The drawing under review shows one solid part. Ordinate dimensions are in mm from its lowest x, y, z. Give positions to 0.01 mm unless a question says otherwise; leave off trailing zeros. Loops run counter-clockwise (first coordinate to the right, second up) from the corner with the lowest first, then second, coordinate; pieces in that order, holes last. Notation, with made-up numbers: (43, -21) - (53, -21) arc R34 cw to (53, 15) - close; hole circle Ø11 at (-31.75, 80.25). An arc over 180 degrees is marked (long way). Write each question's results on one line, items separated by ' | '.
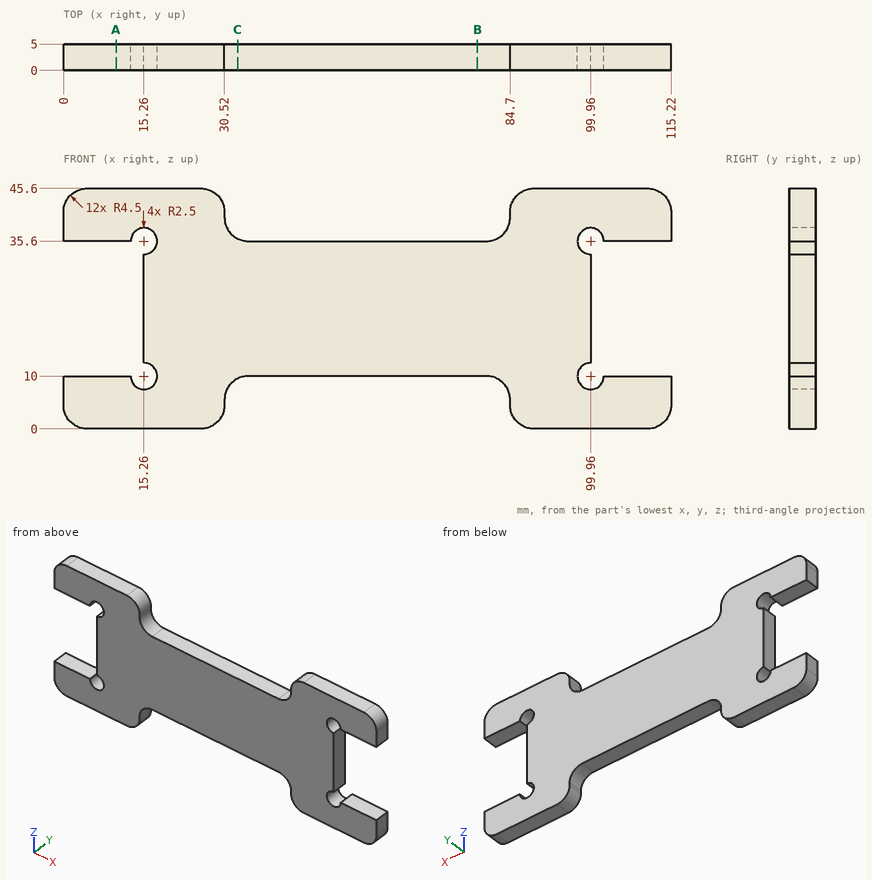
(1) Take a section at A-A on x = 10. Give the boundary of the cut face in (y, z), plus the area to 3 significant figures.
Answers below:
outline: (0, 0) - (5, 0) - (5, 10) - (0, 10) - close; (0, 35.6) - (5, 35.6) - (5, 45.6) - (0, 45.6) - close | area: 100 mm2
(2) Wall thickness on line 1 along Z through (x, y) = (109, 0.65); line 2 along Z through (x, y) = (17.5, 3.4); line 3 along X through (y, z) = (0.8, 14.5): over which ranges is each line inside the solid? List them lowest first. Write a range as from..to.
Answers below:
line 1: 0..10, 35.6..45.6 | line 2: 0..8.89, 11.11..34.49, 36.71..45.6 | line 3: 15.26..99.96
(3) Take a section at B-B on x = 78.5. Give the boundary of the cut face in (y, z), plus the area to 3 significant figures.
Answers below:
outline: (0, 10) - (5, 10) - (5, 35.6) - (0, 35.6) - close | area: 128 mm2
(4) Take a section at C-C on x = 33. Give the boundary of the cut face in (y, z).
Answers below:
outline: (0, 9.52) - (5, 9.52) - (5, 36.08) - (0, 36.08) - close
(5) Insertion check: P1, Ø2.5, axis at x = 111.5, y = 3.5, coming from the -Z side; P2, Ø2.5, axis at y = 3, z = 18.5, coming from the +X side; P3, Ø1.5, axis at y = 2, z = 27, coming from the -X side; P4, Ø1.5, axis at x = 67.5, y = 2, coming from the -Z side. Each pin has a flat end and moves straight along its axis. Give the tip position at first contact, or say it passes through.
Answers below:
P1: z = 0 | P2: x = 99.96 | P3: x = 15.26 | P4: z = 10
